from build123d import *

# Parameters (mm, degrees)
F0_W     = 90
F0_H     = 50
F0_H_2   = 30
F0_R     = 1.55
F0_W_2   = 19
F0_H_3   = 3
F1_DEPTH = 4
F3_DEPTH = 4
F4_W     = 0.5
F4_H     = 20
F5_DEPTH = 0.5


with BuildPart() as f1:
    # F0 (on Front) → F1 (new body)
    with BuildSketch(Plane.XZ):
        Polygon((50.859297, 66.157015), (-49.140703, 66.157015), (-49.140703, -63.842985), (-9.140703, -63.842985), (-9.140703, -83.842985), (10.859297, -83.842985), (10.859297, -63.842985), (50.859297, -63.842985), align=None)
        with Locations((0.859297, -28.842985)):
            Rectangle(F0_W, F0_H, mode=Mode.SUBTRACT)
        with Locations((0.859297, 21.157015)):
            Rectangle(F0_W, F0_H_2, mode=Mode.SUBTRACT)
        with Locations((-26.640703, 41.357015)):
            Circle(F0_R, mode=Mode.SUBTRACT)
        with Locations((0.859297, 57.657015)):
            Rectangle(F0_W_2, F0_H_3, mode=Mode.SUBTRACT)
        with Locations((28.359297, 56.357015)):
            Circle(F0_R, mode=Mode.SUBTRACT)
    extrude(amount=F1_DEPTH)

    # F2 (on face) → F3 (join)
    with BuildSketch(Plane.XY.offset(6.157015)):
        with BuildLine():
            Line((-49.140703, 105), (-49.140703, 0))
            Line((-49.140703, 0), (-29.140703, 0))
            Line((-29.140703, 0), (-29.140703, 105))
            ThreePointArc((-29.140703, 105), (-30.605169, 108.535534), (-34.140703, 110))
            Line((-34.140703, 110), (-44.140703, 110))
            ThreePointArc((-44.140703, 110), (-47.676237, 108.535534), (-49.140703, 105))
        make_face()
        Polygon((-46.854805, 62), (-43.390703, 64), (-39.926602, 62), (-39.926602, 58), (-43.390703, 56), (-46.854805, 58), align=None, mode=Mode.SUBTRACT)
        with BuildLine():
            Line((30.859297, 105), (30.859297, 0))
            Line((30.859297, 0), (50.859297, 0))
            Line((50.859297, 0), (50.859297, 105))
            ThreePointArc((50.859297, 105), (49.394831, 108.535534), (45.859297, 110))
            Line((45.859297, 110), (35.859297, 110))
            ThreePointArc((35.859297, 110), (32.323763, 108.535534), (30.859297, 105))
        make_face()
        Polygon((45.109297, 64), (48.573398, 62), (48.573398, 58), (45.109297, 56), (41.645195, 58), (41.645195, 62), align=None, mode=Mode.SUBTRACT)
    extrude(amount=-F3_DEPTH)

    # F4 (on face) → F5 (cut)
    with BuildSketch(Plane(origin=(0, 0, 0), x_dir=(-1, 0, 0), z_dir=(0, 1, 0))):
        with Locations((-0.859297, -73.842985)):
            Rectangle(F4_W, F4_H)
    extrude(amount=-F5_DEPTH, mode=Mode.SUBTRACT)


solid = f1.part
Work out the finished part from the listing and answer in its coordinate system (mm). A direction names the side the tool comes from. Give positions to 0.01 mm unless a question says otherwise; leave off trailing zeros. Write each loop counter-clockwise with the first axis right and the second up, starting at its lowest first coordinate (ties: lowest second). Pieces come first, ordered by that corner, then holes. Notation, with made-up numbers: M 88.25,45 L 108.25,45 A11 ccw 108.25,54 Z; hole C 63.25,-33 d4. An arc over 180 degrees is marked long. Answer as CSV lines item,"result".
Q1. A tool of negligible diameter and unlimited length cuts with its end or side. For faces 5 (the flat face through (2, -2, 66.157)), 6 (the flat face through (41.645, 60, 4)), 7 (the flat face through (-9.141, -2, -74)), 8 (the flat face through (0, -2, 36.157)), 9 (the flat face through (41, 56, 2.157)), from which of +Z, -Z, +X, -X, +Y, -Y can it reach the whole face along a straight path? Write none if from no direction.
A:
face 5,"+Z, +X, -X, +Y, -Y"
face 6,"+Z, -Z"
face 7,"-Z, -X, +Y, -Y"
face 8,"+Y, -Y"
face 9,"-Z, +X, -X, +Y"
Q2. Given P1, Ø4.5, axis at x = -24.5, y = -2.5, coming from the -Z side; P2, Ø8, axis at x = -29, y = 9.5, coming from the -Z side; P3, Ø4.5, axis at y = -2.5, z = -78, coming from the -X side, each flat-ended and moving along its own axis, determine where each tip first touches the part or whether it passes through.
A:
P1,"stops at z = -63.84"
P2,"stops at z = 2.16"
P3,"stops at x = -9.14"
Q3. A cutting plane is placed at B-B on z = 25. Write down the section's boundary in (x, y), plus the area to 3 significant figures.
A:
outline,"M -49.14,-4 L -44.14,-4 L -44.14,0 L -49.14,0 Z; M 45.86,-4 L 50.86,-4 L 50.86,0 L 45.86,0 Z"
area,"40.0 mm²"
Q4. Find the intervals of material crossed by probe 1 along Y at (x, z) = (21, -3); probe 2 along Z at (x, y) = (-40, 93), in increasing order. Write a range as [from, to].
A:
probe 1,"y = [-4, 0]"
probe 2,"z = [2.16, 6.16]"
Q5. A cutting plane is placed at D-D on y = 82. Write down the section's boundary in (x, z), plus the area to 3 significant figures.
A:
outline,"M -49.14,2.16 L -29.14,2.16 L -29.14,6.16 L -49.14,6.16 Z; M 30.86,2.16 L 50.86,2.16 L 50.86,6.16 L 30.86,6.16 Z"
area,"160 mm²"
Q6. A cutting plane is placed at A-A on x = -18. Write down the section's boundary in (y, z), plus the area to 3 significant figures.
A:
outline,"M -4,-63.84 L 0,-63.84 L 0,-53.84 L -4,-53.84 Z; M -4,-3.84 L 0,-3.84 L 0,6.16 L -4,6.16 Z; M -4,36.16 L 0,36.16 L 0,66.16 L -4,66.16 Z"
area,"200 mm²"
Q7. The mould has two halves that part along X. Classify faces 1 (the flat face through (10.859, -2, -74)), 2 (the cylindrical face through (-47.64, 108.57, 4.19)), 3 (the flat face through (-39, 110, 4)), 4 (the cylindrical face through (-30.57, 108.5, 4.19)): +X half, -X half, draft (parallel to the pull), parting line (faces both ways), or undercut.
A:
face 1,"+X half"
face 2,"-X half"
face 3,"draft"
face 4,"undercut"
Q8. A cutting plane is placed at C-C on x = 7. Write down the section's boundary in (y, z).
A:
outline,"M -4,-83.84 L 0,-83.84 L 0,-53.84 L -4,-53.84 Z; M -4,-3.84 L 0,-3.84 L 0,6.16 L -4,6.16 Z; M -4,36.16 L 0,36.16 L 0,56.16 L -4,56.16 Z; M -4,59.16 L 0,59.16 L 0,66.16 L -4,66.16 Z"
